Could you check a few things on this model? Use its own coordinates, in mm. Round coordinates to 2 decimals unless told otherwise and drop trailing zeros. Loops run counter-clockwise (first coordinate to the right, second up) from the corner with the lowest first, then second, coordinate; pieces in that order, holes last. Notation, with made-up numbers: (12.25, -13.5) -> (30.25, -13.5) arc R24 cw to (30.25, 12.5) -> close; hole circle Ø3 at (86.5, 70). An arc over 180 degrees is marked (long way). Use CSV: the item, a comma, the result in double quotes. Start each with the question number.
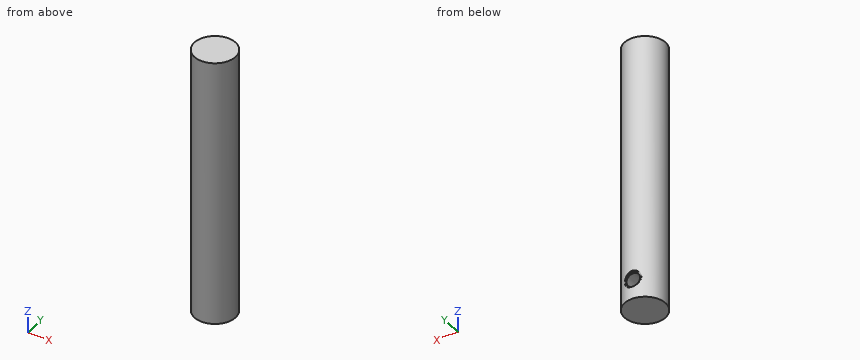
```python
from build123d import *

# Parameters (mm, degrees)
SKETCH_1_W             = 5
SKETCH_1_H             = 65
SKETCH_2_R             = 2
CUT_EXTRUDE_1_DEPTH    = 0.5
HOLE_WIZARD_M4_2_D     = 3.3
HOLE_WIZARD_M4_2_DEPTH = 5
HOLE_WIZARD_M4_2_TIP   = 0.991420021


with BuildPart() as part:
    # 草圖1 → 旋轉1 (revolve)
    with BuildSketch(Plane(origin=(0, 0, 0), x_dir=(1, 0, 0), z_dir=(0, 1, 0))):
        with Locations((2.5, 32.5)):
            Rectangle(SKETCH_1_W, SKETCH_1_H)
    revolve(axis=Axis((0, 0, 16.74665181), (0, 0, -1)))

    # 草圖2 → 除料-伸長1 (cut)
    with BuildSketch(Plane(origin=(0, 5, 0), x_dir=(1, 0, 0), z_dir=(0, 1, 0))):
        with Locations((0, 60)):
            Circle(SKETCH_2_R)
    extrude(amount=-CUT_EXTRUDE_1_DEPTH, mode=Mode.SUBTRACT)

    # M4 螺紋孔2
    with Locations(Plane(origin=(0, 4.5, -60), x_dir=(0, 0, 1), z_dir=(0, 1, 0))):
        with Locations((0, 0)):
            Hole(HOLE_WIZARD_M4_2_D / 2, depth=HOLE_WIZARD_M4_2_DEPTH)
            with Locations((0, 0, -(HOLE_WIZARD_M4_2_DEPTH + HOLE_WIZARD_M4_2_TIP / 2))):  # 118° drill point
                Cone(0, HOLE_WIZARD_M4_2_D / 2, HOLE_WIZARD_M4_2_TIP, mode=Mode.SUBTRACT)


solid = part.part
```
1. Suppose I cut it at A-A (y = 2.25). List the corners of the cut face in (x, z) for me, then the cut area to 3 significant figures.
2. Suppose I cut it at C-C (z = -54). List the corners of the cut face in (x, y) for me, then the cut area to 3 significant figures.
3. Suppose I cut it at D-D (x = 3.75). List the corners of the cut face in (y, z) for me.
4. Suppose I cut it at B-B (x = -4). List the corners of the cut face in (y, z) for me, then the cut area to 3 significant figures.
5. If I drill on L1, parallel to Z at x = 0, y = 4.7; L2, parallel to Z at x = 0, y = 0.95; L3, parallel to X at y = 1.4, z = -60, over which ranges is the centre line in solid material (lowest first)?
6. Will these pins go through, and if not, where does the flat tip stop? pin 1 (2 mm diameter, centred on x = -1.5, z = -10, fed in from -Y); pin 2 (3 mm diameter, centred on y = -2.5, z = -8.5, fed in from +X); pin 3 (6 mm diameter, centred on x = -4, z = -26, fed in from +Y).
Geometry check:
1,outline,"(-4.47, -65) -> (4.47, -65) -> (4.47, 0) -> (-4.47, 0) -> close; hole circle Ø3.3 at (0, -60)"
1,area,"572 mm²"
2,outline,"circle Ø10 at (0, 0)"
2,area,"78.5 mm²"
3,outline,"(-3.31, -65) -> (3.31, -65) -> (3.31, 0) -> (-3.31, 0) -> close"
4,outline,"(-3, -65) -> (3, -65) -> (3, 0) -> (-3, 0) -> close"
4,area,"390 mm²"
5,L1,"z = -65 to -62, -58 to 0"
5,L2,"z = -65 to -61.65, -58.35 to 0"
5,L3,"x = -4.8 to -1.65, 1.65 to 4.8"
6,pin 1,"stops at y = -4.97"
6,pin 2,"stops at x = 4.9"
6,pin 3,"stops at y = 4.9"
